Read the model definition and answer for the solid it produces. Units are mm, in the model's axes. Give positions to 0.01 mm unless a question says otherwise; leave off trailing zeros. Order: outer loops, then holes, each group sorted by start corner. A loop starts at its lowest first (then second) coordinate and runs counter-clockwise, first axis right, second up.
```python
from build123d import *

# Parameters (mm, degrees)
SKETCH1_W           = 100
SKETCH1_H           = 80
SKETCH1_R           = 5
BOSS_EXTRUDE3_DEPTH = 5


with BuildPart() as part:
    # Sketch1 → Boss-Extrude3 (new body)
    with BuildSketch(Plane.XY):
        Rectangle(SKETCH1_W, SKETCH1_H)
        with Locations((-26.18590973, 0)):
            Circle(SKETCH1_R, mode=Mode.SUBTRACT)
        with Locations((0, 26.18590973)):
            Circle(SKETCH1_R, mode=Mode.SUBTRACT)
        with Locations((26.18590973, 0)):
            Circle(SKETCH1_R, mode=Mode.SUBTRACT)
        with Locations((0, -26.18590973)):
            Circle(SKETCH1_R, mode=Mode.SUBTRACT)
    extrude(amount=-BOSS_EXTRUDE3_DEPTH)


solid = part.part
```
1) The part is cut by section C-C on z = -2.6. Determine the outline of the cut face in (x, y).
Final values:
outline: (-50, -40) - (50, -40) - (50, 40) - (-50, 40) - close; hole circle Ø10 at (-26.19, 0); hole circle Ø10 at (0, -26.19); hole circle Ø10 at (0, 26.19); hole circle Ø10 at (26.19, 0)
2) The part is cut by section A-A on y = 0. Determine the outline of the cut face in (x, z).
Final values:
outline: (-50, -5) - (-31.19, -5) - (-31.19, 0) - (-50, 0) - close; (-21.19, -5) - (21.19, -5) - (21.19, 0) - (-21.19, 0) - close; (31.19, -5) - (50, -5) - (50, 0) - (31.19, 0) - close
3) Consider L1, parallel to Y at x = 0, z = -2.35; L2, parallel to Y at x = -3, z = -0.75; L3, parallel to X at y = 25.5, z = -1.35. Determine where each line is inside the solid, lowest interval first.
Final values:
L1: y = -40 to -31.19, -21.19 to 21.19, 31.19 to 40
L2: y = -40 to -30.19, -22.19 to 22.19, 30.19 to 40
L3: x = -50 to -4.95, 4.95 to 50
4) The part is cut by section D-D on y = -27.5. Determine the outline of the cut face in (x, z), and give its area (3 significant figures).
Final values:
outline: (-50, -5) - (-4.82, -5) - (-4.82, 0) - (-50, 0) - close; (4.82, -5) - (50, -5) - (50, 0) - (4.82, 0) - close
area: 452 mm2
5) The part is cut by section B-B on x = 0. Determine the outline of the cut face in (y, z), and give its area (3 significant figures).
Final values:
outline: (-40, -5) - (-31.19, -5) - (-31.19, 0) - (-40, 0) - close; (-21.19, -5) - (21.19, -5) - (21.19, 0) - (-21.19, 0) - close; (31.19, -5) - (40, -5) - (40, 0) - (31.19, 0) - close
area: 300 mm2
6) For a pull along Y with two mould halves and no side action, classify faces 1 (the face through (-1, 1, -5)), 2 (the face through (-1, 40, -2)), 3 (the face through (-3.968, 23.143, -2.465)) as released by +Y, released by -Y, zero draft, split by the parting line, or undercut.
Final values:
face 1: zero draft
face 2: released by +Y
face 3: undercut
